The model under review builds one solid part; all positions refer to its coordinate system, in mm. Round coordinates to 2 decimals unless told otherwise and drop trailing zeros. Order: outer loops, then holes, each group sorted by start corner. A loop starts at its lowest first (then second) coordinate and runs counter-clockwise, first axis right, second up. Notation, with made-up numbers: (66.25, -37.5) -> (98.25, -37.5) arc R13 ccw to (98.25, -14.5) -> close; hole circle Ø4 at (-7.5, 79.25). An arc over 180 degrees is marked (long way). Return JSON: item names as keys, results as strings. Group by question number.
from build123d import *

# Parameters (mm, degrees)
SKETCH1_R           = 3.5
BOSS_EXTRUDE1_DEPTH = 16
BOSS_EXTRUDE2_START = 0.5
BOSS_EXTRUDE2_DEPTH = 0.5
SKETCH3_R           = 0.4
BOSS_EXTRUDE3_DEPTH = 3.5
FILLET2_R           = 0.25
FILLET3_R           = 0.25


with BuildPart() as part:
    # Sketch1 → Boss-Extrude1 (new body)
    with BuildSketch(Plane(origin=(0, 0, 0), x_dir=(1, 0, 0), z_dir=(0, 1, 0))):
        with Locations(Location((0, 0, 0), (0, 0, 270))):
            Circle(SKETCH1_R)
    extrude(amount=BOSS_EXTRUDE1_DEPTH)

    # Sketch2 → Boss-Extrude2 (add)
    with BuildSketch(Plane.XZ.offset(BOSS_EXTRUDE2_START)):
        with BuildLine():
            Line((-0.5, 2.964101615), (0.5, 2.964101615))
            Line((0.5, 2.964101615), (0.5, 3.464101615))
            ThreePointArc((0.5, 3.464101615), (2.474873734, 2.474873734), (3.464101615, 0.5))
            Line((3.464101615, 0.5), (2.964101615, 0.5))
            Line((2.964101615, 0.5), (2.964101615, -0.5))
            Line((2.964101615, -0.5), (3.464101615, -0.5))
            ThreePointArc((3.464101615, -0.5), (2.474873734, -2.474873734), (0.5, -3.464101615))
            Line((0.5, -3.464101615), (0.5, -2.964101615))
            Line((0.5, -2.964101615), (-0.5, -2.964101615))
            Line((-0.5, -2.964101615), (-0.5, -3.464101615))
            ThreePointArc((-0.5, -3.464101615), (-2.474873734, -2.474873734), (-3.464101615, -0.5))
            Line((-3.464101615, -0.5), (-2.964101615, -0.5))
            Line((-2.964101615, -0.5), (-2.964101615, 0.5))
            Line((-2.964101615, 0.5), (-3.464101615, 0.5))
            ThreePointArc((-3.464101615, 0.5), (-2.474873734, 2.474873734), (-0.5, 3.464101615))
            Line((-0.5, 3.464101615), (-0.5, 2.964101615))
        make_face()
    extrude(amount=-BOSS_EXTRUDE2_DEPTH)

    # Sketch3 → Boss-Extrude3 (add)
    with BuildSketch(Plane(origin=(0, 16, 0), x_dir=(1, 0, 0), z_dir=(0, 1, 0))):
        with Locations(Location((0, 0, 0), (0, 0, 270))):
            Circle(SKETCH3_R)
    extrude(amount=BOSS_EXTRUDE3_DEPTH)

    # Fillet2
    fillet2_edges = [part.edges().sort_by_distance(p)[0] for p in [
        (0, 16, -3.5),
    ]]
    fillet(fillet2_edges, radius=FILLET2_R)

    # Fillet3
    fillet3_edges = [part.edges().sort_by_distance(p)[0] for p in [
        (0, 19.5, -0.4),
    ]]
    fillet(fillet3_edges, radius=FILLET3_R)


solid = part.part
Item 1: Insertion check: pin 1 Ø1 at (y, z) = (5.5, -1.5) entering from -X; pin 2 Ø1 at (x, z) = (-2, -2) entering from +Y; pin 3 Ø0.6 at (y, z) = (0, -3.5) entering from -X. Each pin has a flat end and moves straight along its axis. Give the tip position at first contact, or say it passes through.
Item 2: Wall thickness on line 1 along Y through (x, z) = (-2, 0.5); line 2 along X through (y, z) = (4.75, -0.5); line 3 along Z through (x, y) = (1.5, 6.5): over which ranges is each line inside the solid? List them lowest first.
Item 3: Consider section A-A on y = 17.5. State the section outline as (x, z) points, plus the area to 3 significant figures.
Values:
{
 "1": {"pin 1": "x = -3.35", "pin 2": "y = 16", "pin 3": "x = -1.42"},
 "2": {"line 1": "-0.5 to 16", "line 2": "-3.46 to 3.46", "line 3": "-3.16 to 3.16"},
 "3": {"outline": "circle Ø0.8 at (0, 0)", "area": "0.503 mm^2"}
}
